from build123d import *

# Parameters (mm, degrees)
F1_DEPTH = 1.5875


with BuildPart() as f1:
    # F0 (on Top) → F1 (new body)
    with BuildSketch(Plane.XY):
        with BuildLine():
            ThreePointArc((-3.175, 0), (-2.245064, 2.245064), (0, 3.175))
            Line((0, 3.175), (-41.275, 4.7625))
            Line((-41.275, 4.7625), (-50.8, 0))
            Line((-50.8, 0), (-3.175, 0))
        make_face()
        with BuildLine():
            ThreePointArc((0, -3.175), (2.245064, -2.245064), (3.175, 0))
            ThreePointArc((3.175, 0), (2.245064, 2.245064), (0, 3.175))
            ThreePointArc((0, 3.175), (-2.245064, 2.245064), (-3.175, 0))
            ThreePointArc((-3.175, 0), (-2.245064, -2.245064), (0, -3.175))
        make_face()
        with BuildLine():
            Line((-41.275, -4.7625), (0, -3.175))
            ThreePointArc((0, -3.175), (-2.245064, -2.245064), (-3.175, 0))
            Line((-3.175, 0), (-50.8, 0))
            Line((-50.8, 0), (-41.275, -4.7625))
        make_face()
    extrude(amount=F1_DEPTH)


with BuildPart() as f2_1:
    # F2: copy of F1
    add(f1.part)


solid = f1.part
Work out the finished part from the listing and answer in its coordinate system (mm). Round coordinates to 2 decimals unless told otherwise and drop trailing zeros. Write each loop counter-clockwise with the first axis right and the second up, starting at its lowest first coordinate (ties: lowest second). Pieces come first, ordered by that corner, then holes.
1) Straight lines are drawn through the part: line 1 (Y direction, x = -33, z = 1.45); line 2 (Y direction, x = -48.5, z = 0.25); line 3 (X direction, y = -0.5, z = 0.6). For each, find the intervals that lie inside material, in ascending order.
2) A cutting plane is placed at B-B (x = -32). Give the vertices of the cut face in (y, z), plus the area to 3 significant figures.
3) A cutting plane is placed at C-C (y = 1.75). Give the vertices of the cut face in (x, z).
Completed:
1. line 1: y = -4.44 to 4.44
1. line 2: y = -1.15 to 1.15
1. line 3: x = -49.8 to 3.14
2. outline: (-4.41, 0) - (4.41, 0) - (4.41, 1.59) - (-4.41, 1.59) - close
2. area: 14.0 mm2
3. outline: (-47.3, 0) - (2.65, 0) - (2.65, 1.59) - (-47.3, 1.59) - close
